Can you work these out from the model? Positions are in its coordinate system, mm. A direction names the side the tool comes from. Give positions to 0.01 mm unless a question says otherwise; leave off trailing zeros. Write each loop counter-clockwise with the first axis right and the second up, starting at its lowest first coordinate (ties: lowest second). Pieces come first, ordered by that corner, then holes.
```python
from build123d import *

# Parameters (mm, degrees)
BOSS_EXTRUDE1_DEPTH = 2.794
SKETCH2_R           = 0.9525
SKETCH2_R_2         = 3.302
CUT_EXTRUDE1_DEPTH  = 63.960241994
FILLET2_R           = 2.54


with BuildPart() as part:
    # Sketch1 → Boss-Extrude1 (new body)
    with BuildSketch(Plane(origin=(0, 0, 0), x_dir=(1, 0, 0), z_dir=(0, 1, 0))):
        Polygon((59.944, 0), (21.844, 0), (9.144, -3.175), (5.969, -3.175), (5.969, 0), (3.175, 0), (3.175, -3.175), (0, -3.175), (0, 3.175), (8.362279277, 3.175), (21.844, 6.545430181), (28.194, 6.545430181), (28.194, 19.05), (59.944, 19.05), align=None)
    extrude(amount=BOSS_EXTRUDE1_DEPTH)

    # Sketch2 → Cut-Extrude1 (cut, through all)
    with BuildSketch(Plane(origin=(0, 2.794, 0), x_dir=(1, 0, 0), z_dir=(0, 1, 0))):
        with Locations(Location((56.769, 3.175, 0), (0, 0, 270))):
            Circle(SKETCH2_R)
        with Locations(Location((35.769, 3.175, 0), (0, 0, 270))):
            Circle(SKETCH2_R)
        with Locations(Location((53.594, 12.7, 0), (0, 0, 270))):
            Circle(SKETCH2_R_2)
        with Locations(Location((38.944, 12.7, 0), (0, 0, 270))):
            Circle(SKETCH2_R_2)
    extrude(amount=-CUT_EXTRUDE1_DEPTH, mode=Mode.SUBTRACT)

    # Fillet2
    fillet2_edges = [part.edges().sort_by_distance(p)[0] for p in [
        (59.944, 1.397, 0),
        (28.194, 1.397, -19.05),
        (59.944, 1.397, -19.05),
    ]]
    fillet(fillet2_edges, radius=FILLET2_R)


solid = part.part
```
1) Suppose I cut it at D-D on x = 26. Write out the boundary of the cut face in (y, z), plus the area to 3 significant figures.
Values follow:
outline: (0, -6.55) - (2.79, -6.55) - (2.79, 0) - (0, 0) - close
area: 18.3 mm2
2) If we mould it in two halves opening along X, with no side actions, what happens to faces 4 (the face through (40, 1, 0)), 5 (the face through (28.96, 1.42, -18.33)), 6 (the face through (5, 1, 0))? For each: +X half, -X half, draft (parallel to the pull), parting line (faces both ways), or undercut.
Values follow:
face 4: draft
face 5: -X half
face 6: undercut
3) For pin 1 Ø1.4 at (x, y) = (5, 1) entering from -Z (3 decimals); pin 2 Ø1.4 at (y, z) = (1.5, -11) entering from -X; pin 3 Ø1 at (x, y) = (53.5, 1) entering from +Z, each with a flat end and sliding along its axis, tell me the tip position at first contact or that it passes through.
Values follow:
pin 1: stops at z = -3.175
pin 2: stops at x = 28.19
pin 3: stops at z = 0
4) Suppose I cut it at B-B on y = 0.8. State how many separate pieces and enclosed holes the cut face has, plus the area to 3 significant figures.
Values follow:
separate pieces: 1
enclosed holes: 4
area: 700 mm2
5) Suppose I cut it at C-C on z = -7.5. Write out the boundary of the cut face in (x, y).
Values follow:
outline: (28.19, 0) - (59.94, 0) - (59.94, 2.79) - (28.19, 2.79) - close
6) Suppose I cut it at A-A on z = -12.7. Write out the boundary of the cut face in (x, y), plus the area to 3 significant figures.
Values follow:
outline: (28.19, 0) - (35.64, 0) - (35.64, 2.79) - (28.19, 2.79) - close; (42.25, 0) - (50.29, 0) - (50.29, 2.79) - (42.25, 2.79) - close; (56.9, 0) - (59.94, 0) - (59.94, 2.79) - (56.9, 2.79) - close
area: 51.8 mm2
7) Please list where these lines run through material, in increasing order: L1, parallel to X at y = 0.7, z = -12.7; L2, parallel to X at y = 0.75, z = -13.25; L3, parallel to Z at x = 56.5, y = 1.55.
Values follow:
L1: x = 28.19 to 35.64, 42.25 to 50.29, 56.9 to 59.94
L2: x = 28.19 to 35.69, 42.2 to 50.34, 56.85 to 59.94
L3: z = -19.05 to -14.27, -11.13 to -4.09, -2.26 to 0
8) For faces 1 (the face through (37, 0, -8)), 2 (the face through (3.175, 1, 2)), 3 (the face through (28.194, 1, -11)), which set-ups out of +Z, -Z, +X, -X, +Y, -Y let a thin tool reach every point of the face, with its end or its side?
Values follow:
face 1: +Z, -Z, +X, -X, -Y
face 2: +Z, +Y, -Y
face 3: -Z, -X, +Y, -Y
